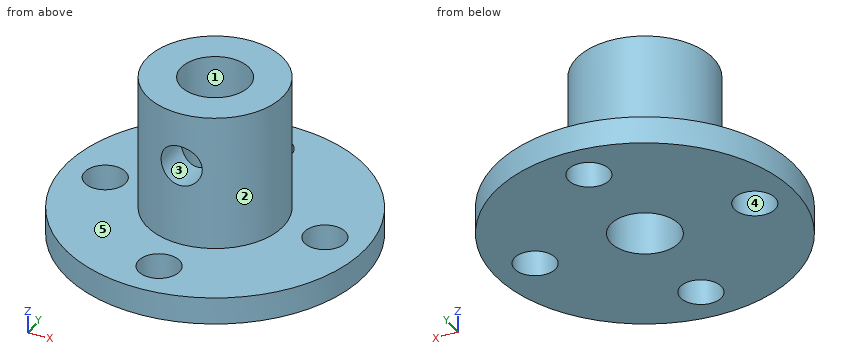
from build123d import *

# Parameters (mm, degrees)
SKETCH2_R           = 10.999999971
BOSS_EXTRUDE1_DEPTH = 2
SKETCH3_R           = 5
BOSS_EXTRUDE2_DEPTH = 10
SKETCH4_R           = 2.5
CUT_EXTRUDE1_DEPTH  = 20.646882672
SKETCH5_R           = 1.500000048
CUT_EXTRUDE2_DEPTH  = 10
SKETCH6_R           = 1.5
CUT_EXTRUDE3_DEPTH  = 19.493242028
CIRPATTERN1_COUNT   = 4


with BuildPart() as part:
    # Sketch2 → Boss-Extrude1 (new body)
    with BuildSketch(Plane.XY):
        Circle(SKETCH2_R)
    extrude(amount=BOSS_EXTRUDE1_DEPTH)

    # Sketch3 → Boss-Extrude2 (add)
    with BuildSketch(Plane.XY.offset(2)):
        Circle(SKETCH3_R)
    extrude(amount=BOSS_EXTRUDE2_DEPTH)

    # Sketch4 → Cut-Extrude1 (cut, through all)
    with BuildSketch(Plane.XY.offset(12)):
        Circle(SKETCH4_R)
    extrude(amount=-CUT_EXTRUDE1_DEPTH, mode=Mode.SUBTRACT)

    # Sketch5 → Cut-Extrude2 (cut)
    with BuildSketch(Plane(origin=(0, 0, 0), x_dir=(1, 0, 0), z_dir=(0, 1, 0))):
        with Locations(Location((0, -8, 0), (0, 0, 270))):
            Circle(SKETCH5_R)
    extrude(amount=-CUT_EXTRUDE2_DEPTH, mode=Mode.SUBTRACT)

    # Sketch6 → Cut-Extrude3 (cut, through all)
    with BuildSketch(Plane.XY.offset(2)):
        with Locations((0, 8)):
            Circle(SKETCH6_R)
    cut_extrude3 = extrude(amount=-CUT_EXTRUDE3_DEPTH, mode=Mode.SUBTRACT)

    # CirPattern1: Cut-Extrude3 ×4 about axis
    cirpattern1_axis = Axis((0, 0, 0), (0, 0, 1))
    for i in range(1, CIRPATTERN1_COUNT):
        add(cut_extrude3.rotate(cirpattern1_axis, i * 360 / CIRPATTERN1_COUNT), mode=Mode.SUBTRACT)


solid = part.part
Model file for the job. Use its own axes, mm. Face numbers are marked on the shaded views. A direction names the side the tool comes from. Round coordinates to 2 decimals unless told otherwise and drop trailing zeros. Order: outer loops, then holes, each group sorted by start corner. A loop starts at its lowest first (then second) coordinate and runs counter-clockwise, first axis right, second up. Notation, with made-up numbers: M -38,84 L -23,84 A28 cw -23,120 Z; hole C 27.25,-21 d8. An arc over 180 degrees is marked long. Write each question's results on one line, items separated by ' | '. Start each with the question number.
(1) Saw through at C-C, the plane x = -8. Give the cut face in (y, z), then the cut area to 3 significant figures.
(2) Which spindle directions (+Z, -Z, +X, -X, +Y, -Y) get a long thin tool onto all of the face, cutting with end or side? Do the marked faces 4 and 5. Say none if no direction does.
(3) Saw through at B-B, the plane y = 0. Give the cut face in (x, z).
(4) Saw through at D-D, the plane y = -9. Give the cut face in (x, z).
(5) Two-plate mould, pull along Y, no slides. Class the marked faces 1, 2 and 3: pulls with the +Y half, pulls with the -Y half, needs draft (parallel to the pull), parting line crosses it, or undercut.
(6) Drop flat-ended pins along their axis: pin 1 (4 mm diameter, centred on x = 0, y = -8, fed in from +Z); pin 2 (1.5 mm diameter, centred on x = 3.5, z = 2, fed in from +Y); pin 3 (2.5 mm diameter, centred on x = 0, z = 8, fed in from +Y). Give the stop position or say it passes through.
(7) Saw through at A-A, the plane x = 0. Give the cut face in (y, z).
(8) Probe probe 1 along Z at (x, y) = (4.25, -9); probe 2 along Y at (x, z) = (2, 8.5); probe 3 along X at (y, z) = (1, 6). List the from-to ranges inside material, lowest first. Write a range as from..to.
Established:
1) outline: M -7.55,0 L -1.5,0 L -1.5,2 L -7.55,2 Z; M 1.5,0 L 7.55,0 L 7.55,2 L 1.5,2 Z | area: 24.2 mm^2
2) face 4: +Z, -Z | face 5: +Z
3) outline: M -11,0 L -9.5,0 L -9.5,2 L -11,2 Z; M -6.5,0 L -2.5,0 L -2.5,12 L -5,12 L -5,2 L -6.5,2 Z; M 2.5,0 L 6.5,0 L 6.5,2 L 5,2 L 5,12 L 2.5,12 Z; M 9.5,0 L 11,0 L 11,2 L 9.5,2 Z
4) outline: M -6.32,0 L -1.12,0 L -1.12,2 L -6.32,2 Z; M 1.12,0 L 6.32,0 L 6.32,2 L 1.12,2 Z
5) face 1: undercut | face 2: parting line crosses it | face 3: needs draft
6) pin 1: stops at z = 2 | pin 2: stops at y = 10.65 | pin 3: stops at y = 5
7) outline: M -11,0 L -9.5,0 L -9.5,2 L -11,2 Z; M -6.5,0 L -2.5,0 L -2.5,6.5 L -5,6.5 L -5,2 L -6.5,2 Z; M -5,9.5 L -2.5,9.5 L -2.5,12 L -5,12 Z; M 2.5,0 L 6.5,0 L 6.5,2 L 5,2 L 5,12 L 2.5,12 Z; M 9.5,0 L 11,0 L 11,2 L 9.5,2 Z
8) probe 1: z = 0..2 | probe 2: y = -4.58..-1.5, 1.5..4.58 | probe 3: x = -4.9..-2.29, 2.29..4.9
